Autodesk Inventor part; units mm, degrees
ref_plane "YZ Plane" through (0, 0, 0) normal (1, 0, 0) x (0, 1, 0)
ref_plane "XZ Plane" through (0, 0, 0) normal (0, 1, 0) x (-1, 0, 0)
ref_plane "XY Plane" through (0, 0, 0) normal (0, 0, 1) x (1, 0, 0)
sketch "Sketch1" plane through (0, 0, 0) normal (0, 1, 0) x (-1, 0, 0)
  line L0 (-240, 168.915) -> (240, 168.915)
  line L1 (240, 168.915) -> (240, -168.915)
  line L2 (240, -168.915) -> (-240, -168.915)
  line L3 (-240, -168.915) -> (-240, 168.915)
  line L4 (-240, 168.915) -> (240, -168.915) construction
  line L5 (240, 168.915) -> (-240, -168.915) construction
  point P0 (0, 0)
  dimension "d0" = 480
  dimension "d1" = 337.83
extrude "Extrusion1" add sketch "Sketch1" along normal blind 5
sketch "Sketch2" plane through (0, 5, 0) normal (0, 1, 0) x (1, 0, 0)
  line L0 (240, -168.915) -> (240, 168.915)
  line L1 (240, -168.915) -> (240, -148.915)
  line L2 (240, -148.915) -> (225, -148.915)
  line L3 (-240, -168.915) -> (240, -168.915)
  line L4 (225, -168.915) -> (225, -160.915)
  line L5 (225, -168.915) -> (233, -168.915) construction
  line L6 (225, -148.915) -> (225, -160.915)
  line L7 (225, -160.915) -> (193, -160.915)
  line L8 (193, -160.915) -> (193, -168.915)
  line L9 (193, -168.915) -> (240, -168.915)
  line L10 (240, 0) -> (160.3142, 0)
  line L11 (240, 168.915) -> (240, 148.915)
  line L12 (240, 148.915) -> (225, 148.915)
  line L13 (225, 168.915) -> (225, 160.915)
  line L14 (225, 168.915) -> (233, 168.915) construction
  line L15 (225, 148.915) -> (225, 160.915)
  line L16 (225, 160.915) -> (193, 160.915)
  line L17 (193, 160.915) -> (193, 168.915)
  line L18 (193, 168.915) -> (240, 168.915)
  point P0 (0, 0)
  dimension "d4" = 20
  dimension "d5" = 15
  dimension "d6" = 8
  dimension "d7" = 90
  dimension "d8" = 12
  dimension "d9" = 32
extrude "Extrusion2" cut sketch "Sketch2" against normal blind 5
sketch "Sketch4" plane through (0, 5, 0) normal (0, 1, 0) x (1, 0, 0)
  line L0 (-240, -168.915) -> (193, -168.915)
  line L1 (-240, -168.915) -> (-200, -168.915)
  line L2 (-200, -168.915) -> (-200, -160.183)
  circle A0 centre (-200, -160.183) radius 2.75
  circle A1 centre (-100, -160.183) radius 2.75
  circle A2 centre (0, -160.183) radius 2.75
  circle A3 centre (100, -160.183) radius 2.75
  line L3 (193, 168.915) -> (-240, 168.915)
  line L4 (-240, 168.915) -> (-180, 168.915)
  line L5 (-180, 168.915) -> (-180, 160.183)
  circle A4 centre (-180, 160.183) radius 2.75
  circle A5 centre (-80, 160.183) radius 2.75
  circle A6 centre (20, 160.183) radius 2.75
  circle A7 centre (120, 160.183) radius 2.75
  point P0 (0, 0)
  dimension "d14" = 40
  dimension "d15" = 8.732
  dimension "d16" = 5.5
  dimension "d19" = 100
  dimension "d24" = 60
  dimension "d25" = 8.732
  dimension "d26" = 5.5
  dimension "d29" = 100
extrude "Extrusion3" cut sketch "Sketch4" against normal blind 10
sketch "Sketch5" plane through (0, 5, 0) normal (0, 1, 0) x (1, 0, 0)
  line L0 (193, 168.915) -> (-240, 168.915)
  line L1 (-240, 168.915) -> (240, 168.915)
  line L2 (240, 168.915) -> (240, -170.085)
  line L3 (240, -170.085) -> (-240, -170.085)
  line L4 (-240, -170.085) -> (-240, 168.915)
  point P0 (0, 0)
  dimension "d36" = 480
  dimension "d37" = 339
sketch "Sketch8" plane through (0, 5, 0) normal (0, 1, 0) x (1, 0, 0)
  line L0 (193, 160.915) -> (225, 160.915)
  line L1 (225, 160.915) -> (190, 160.915)
  line L2 (190, 160.915) -> (190, 140.915)
  line L3 (190, 140.915) -> (225, 140.915)
  line L4 (225, 140.915) -> (225, 160.915)
  point P0 (0, 0)
  dimension "d38" = 35
  dimension "d39" = 20
extrude "Extrusion4" cut sketch "Sketch8" against normal blind 10
sketch "Sketch9" plane through (0, 5, 0) normal (0, 1, 0) x (1, 0, 0)
  circle A0 centre (115, 98.915) radius 2
  line L0 (193, 168.915) -> (-240, 168.915)
  line L1 (240, -148.915) -> (240, 148.915)
  circle A1 centre (115, 48.915) radius 2
  circle A2 centre (-35, 98.915) radius 2
  circle A3 centre (-35, 48.915) radius 2
  line L2 (-35, 98.915) -> (-75, 98.915)
  line L3 (-35, 98.915) -> (5, 98.915) construction
  line L4 (-75, 98.915) -> (-75, 83.915)
  line L5 (-75, 83.915) -> (-75, 98.915)
  line L6 (-75, 98.915) -> (-104, 98.915)
  line L7 (-104, 98.915) -> (-104, 48.915)
  line L8 (-104, 48.915) -> (-75, 48.915)
  line L9 (-75, 48.915) -> (-75, 98.915)
  line L10 (-104, 73.915) -> (-109.5, 73.915)
  line L11 (-75, 73.915) -> (-69.5, 73.915)
  circle A4 centre (-69.5, 73.915) radius 1.75
  circle A5 centre (-109.5, 73.915) radius 1.75
  circle A6 centre (115, -78.915) radius 1.75
  line L12 (-240, -168.915) -> (193, -168.915)
  circle A7 centre (57, -78.915) radius 1.75
  circle A8 centre (115, -29.915) radius 1.75
  circle A9 centre (57, -29.915) radius 1.75
  point P0 (0, 0)
  dimension "d42" = 4
  dimension "d43" = 70
  dimension "d44" = 125
  dimension "d47" = 50
  dimension "d50" = 150
  dimension "d53" = 40
  dimension "d54" = 180
  dimension "d55" = 15
  dimension "d56" = 15
  dimension "d57" = 29
  dimension "d58" = 50
  dimension "d59" = 5.5
  dimension "d60" = 5.5
  dimension "d61" = 3.5
  dimension "d62" = 3.5
  dimension "d63" = 3.5
  dimension "d64" = 90
  dimension "d65" = 125
  dimension "d68" = 58
  dimension "d71" = 49
extrude "Extrusion5" cut sketch "Sketch9" against normal blind 10
properties part number "Acrylic_Panel_Mounts"
For this review, take the finished solid that the model builds, in its own axes (mm). Coordinates: 2 decimals unless noted, no trailing zeros. Answer as CSV lines item,"result". Start each with the question number.
1) Add section A-A (y = 2.8). Count the separate pieces of the cut face and the enclosed holes in it, then the cut area to 3 significant figures.
2) To check wall thickness, follow line 1 along Z through (x, y) = (-80, 2.15) (3 decimals); line 2 along Z through (x, y) = (-77, 4.4) (3 decimals); line 3 along Z through (x, y) = (-35, 2.2) (3 decimals). State the ranges of each line that lie inside material, in increasing order. Write a range as [from, to].
3) Insertion check: P1, Ø1.5, axis at y = 2, z = -163, coming from the +X side; P2, Ø5, axis at x = 0, z = 160.183, coming from the +Y side; P3, Ø2.5, axis at y = 1.5, z = 157.5, coming from the +X side; P4, Ø2.5, axis at x = 235.5, y = 3.5, coming from the -Z side (3 decimals). Each pin has a flat end and moves straight along its axis. Give the tip position at first contact, or say it passes through.
Result:
1,separate pieces,"1"
1,enclosed holes,"19"
1,area,"159,000 mm^2"
2,line 1,"[-168.915, -162.933], [-157.433, -98.915], [-48.915, 168.915]"
2,line 2,"[-168.915, -98.915], [-48.915, 168.915]"
2,line 3,"[-168.915, -100.915], [-96.915, -50.915], [-46.915, 168.915]"
3,P1,"x = 193"
3,P2,"through"
3,P3,"x = 225"
3,P4,"z = -148.915"
